Input: part model. Units: mm. Frame: model coordinates. Coordinates: 2 decimals unless noted, no trailing zeros. Loops run counter-clockwise (first coordinate to the right, second up) from the corner with the lowest first, then second, coordinate; pieces in that order, holes last. Notation, with made-up numbers: (-1, -14) -> (44, -14) arc R16 cw to (44, 17) -> close; hole circle Ø7 at (-13, 21). An arc over 180 degrees is marked (long way). Answer as a JSON object with one key per item and string values.
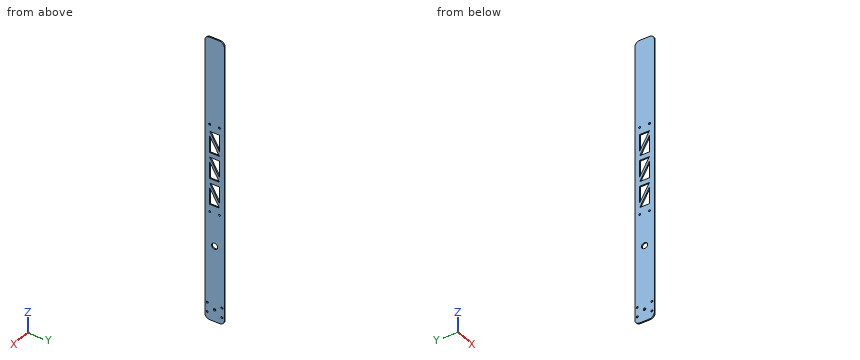
from build123d import *

# Parameters (mm, degrees)
SKETCH1_R           = 7.9629
SKETCH1_R_2         = 3.175
SKETCH1_R_3         = 2.5527
BOSS_EXTRUDE1_DEPTH = 3.175


with BuildPart() as part:
    # Sketch1 → Boss-Extrude1 (new body)
    with BuildSketch(Plane(origin=(0, 0, 0), x_dir=(0, 0, -1), z_dir=(1, 0, 0))):
        with BuildLine():
            Line((177.8, 38.1), (177.8, 12.7))
            ThreePointArc((177.8, 12.7), (174.080256121, 3.719743879), (165.1, 0))
            Line((165.1, 0), (-571.5, 0))
            ThreePointArc((-571.5, 0), (-580.480256121, 3.719743879), (-584.2, 12.7))
            Line((-584.2, 12.7), (-584.2, 38.1))
            ThreePointArc((-584.2, 38.1), (-580.480256121, 47.080256121), (-571.5, 50.8))
            Line((-571.5, 50.8), (165.1, 50.8))
            ThreePointArc((165.1, 50.8), (174.080256121, 47.080256121), (177.8, 38.1))
        make_face()
        with Locations((-25.4, 25.4)):
            Circle(SKETCH1_R, mode=Mode.SUBTRACT)
        with Locations((146.05, 25.4)):
            Circle(SKETCH1_R_2, mode=Mode.SUBTRACT)
        with Locations((-349.25, 38.1)):
            Circle(SKETCH1_R_3, mode=Mode.SUBTRACT)
        with Locations((-349.25, 12.7)):
            Circle(SKETCH1_R_3, mode=Mode.SUBTRACT)
        with Locations((-114.3, 38.1)):
            Circle(SKETCH1_R_3, mode=Mode.SUBTRACT)
        with Locations((-114.3, 12.7)):
            Circle(SKETCH1_R_3, mode=Mode.SUBTRACT)
        with Locations((133.35, 44.45)):
            Circle(SKETCH1_R_3, mode=Mode.SUBTRACT)
        with Locations((158.75, 44.45)):
            Circle(SKETCH1_R_3, mode=Mode.SUBTRACT)
        with Locations((158.75, 6.35)):
            Circle(SKETCH1_R_3, mode=Mode.SUBTRACT)
        with Locations((133.35, 6.35)):
            Circle(SKETCH1_R_3, mode=Mode.SUBTRACT)
        Polygon((-190.5, 38.1), (-146.05, 38.1), (-190.5, 12.7), align=None, mode=Mode.SUBTRACT)
        Polygon((-133.35, 38.1), (-133.35, 12.7), (-177.8, 12.7), align=None, mode=Mode.SUBTRACT)
        Polygon((-203.2, 12.7), (-203.2, 38.1), (-247.65, 12.7), align=None, mode=Mode.SUBTRACT)
        Polygon((-215.9, 38.1), (-260.35, 12.7), (-260.35, 38.1), align=None, mode=Mode.SUBTRACT)
        Polygon((-273.05, 38.1), (-273.05, 12.7), (-317.5, 12.7), align=None, mode=Mode.SUBTRACT)
        Polygon((-330.2, 12.7), (-330.2, 38.1), (-285.75, 38.1), align=None, mode=Mode.SUBTRACT)
    extrude(amount=BOSS_EXTRUDE1_DEPTH)


solid = part.part
1. Line query: line 1 along Y through (x, z) = (1, 114.3); line 2 along Z through (x, y) = (0.75, 38.5); line 3 along Z through (x, y) = (0.2, 8.5). Output: solid intervals per line, ascending.
Reply:
{"line 1": "y = 0 to 10.15, 15.25 to 35.55, 40.65 to 50.8", "line 2": "z = -177.79 to 111.78, 116.82 to 346.73, 351.77 to 584.19", "line 3": "z = -177.09 to -160.13, -157.37 to -134.73, -131.97 to 583.49"}
2. Section query B-B (x = 0.9). Count the separate pieces of the cut face and the enclosed holes in it, plus the area to 3 significant figures.
Reply:
{"separate pieces": "1", "enclosed holes": "16", "area": "34,800 mm2"}
3. Section query A-A (z = 25.4). Return loops of the section in (x, y) (3 decimals).
Reply:
{"outline": "(0, 0) -> (3.175, 0) -> (3.175, 17.437) -> (0, 17.437) -> close; (0, 33.363) -> (3.175, 33.363) -> (3.175, 50.8) -> (0, 50.8) -> close"}
4. Pin query (flat end, axial travel): P1, Ø1, axis at x = 1, y = 9, coming from the +Z side; P2, Ø1, axis at x = 1, y = 6, coming from the +Z side. Return the tip coordinate at first contact, or that it passes through.
Reply:
{"P1": "stops at z = 583.79", "P2": "stops at z = 582.58"}
